Solid Edge part; units mm, degrees
sketch "Sketch1" plane through (0, 0, 0) normal (0, 0, 1) x (1, 0, 0)
  line L0 (-12.6, 6) -> (13.6, 6)
  line L1 (13.6, 6) -> (13.6, 5)
  line L2 (13.6, 5) -> (12.6, 5)
  line L3 (12.6, 5) -> (12.6, -5)
  line L4 (12.6, -5) -> (13.6, -5)
  line L5 (13.6, -5) -> (13.6, -6)
  line L6 (13.6, -6) -> (12.6, -6)
  line L7 (12.6, -6) -> (-12.6, -6)
  line L8 (-12.6, -6) -> (-12.6, 6)
  dimension "D1" = 13.6
  dimension "D2" = 12.6
  dimension "D3" = 12.6
extrude "Protrusion1" add sketch "Sketch1" along normal mid plane 10
sketch "Sketch2" plane through (-12.6, 0, 0) normal (-1, 0, 0) x (0, -1, 0)
  line L0 (-1.118, 1) -> (1.118, 1)
  arc A0 (1.118, 1) -> (-1.118, 1) centre (0, 0) cw
extrude "Extrusionsausprägung_2" add sketch "Sketch2" along normal blind 10
sketch "Sketch3" plane through (0.5, -6, 0) normal (0, -1, 0) x (1, 0, 0)
  line L0 (12.1, 5) -> (12.1, 0.5)
  line L1 (12.1, 0.5) -> (14.7225, 0.5)
  line L2 (14.7225, 0.5) -> (14.7225, -0.5)
  line L3 (14.7225, -0.5) -> (12.1, -0.5)
  line L4 (12.1, -0.5) -> (12.1, -5)
  line L5 (12.1, -5) -> (16.9728, -5)
  line L6 (16.9728, -5) -> (16.9728, 5)
  line L7 (16.9728, 5) -> (12.1, 5)
  dimension "D1" = 14.7225
extrude "Extrusionsausschnitt_1" cut sketch "Sketch3" against normal blind 24
Part model, mm, in its own coordinate system. A direction names the side the tool comes from. Coordinates: 2 decimals unless noted, no trailing zeros. Order: outer loops, then holes, each group sorted by start corner. A loop starts at its lowest first (then second) coordinate and runs counter-clockwise, first axis right, second up. Notation, with made-up numbers: M 62.5,33.5 L 97.5,33.5 A31 ccw 97.5,58.5 Z; hole C 27,37 d11. An arc over 180 degrees is marked long. Use a Markdown table: item, result.
(1) Flat gauge pins, fed straight in: pin 1 (3 mm diameter, centred on y = 0, z = -2, fed in from +X); pin 2 (4 mm diameter, centred on x = -15, z = -1, fed in from +Y); pin 3 (0.7 mm diameter, centred on x = -17, y = 0, fed in from +Z). Where does each tip first touch, or does it go through?
A:
| item | result |
|---|---|
| pin 1 | stops at x = 12.6 |
| pin 2 | stops at y = 1.5 |
| pin 3 | stops at z = 1 |
(2) Cut at A-A on z = 0. Write the cut outline in (x, y).
A:
| item | result |
|---|---|
| outline | M -22.6,-1.5 L -12.6,-1.5 L -12.6,-6 L 13.6,-6 L 13.6,-5 L 12.6,-5 L 12.6,5 L 13.6,5 L 13.6,6 L -12.6,6 L -12.6,1.5 L -22.6,1.5 Z |
(3) Probe L1, parallel to X at y = 1, z = -1; L2, parallel to X at y = -3.25, z = 3.25; L3, parallel to Z at x = -20, y = -0.5. List the from-to ranges inside material, lowest first.
A:
| item | result |
|---|---|
| L1 | x = -22.6 to 12.6 |
| L2 | x = -12.6 to 12.6 |
| L3 | z = -1.41 to 1 |
(4) Cut at B-B on y = 0. Write the cut outline in (x, z).
A:
| item | result |
|---|---|
| outline | M -22.6,-1.5 L -12.6,-1.5 L -12.6,-5 L 12.6,-5 L 12.6,5 L -12.6,5 L -12.6,1 L -22.6,1 Z |
(5) Cut at D-D on z = 1.5. Write the cut outline in (x, y), then the cut area to 3 significant figures.
A:
| item | result |
|---|---|
| outline | M -12.6,-6 L 12.6,-6 L 12.6,6 L -12.6,6 Z |
| area | 302 mm^2 |
(6) Pull direction Y, two halves, no side cores. Call faces 5 (the flat face through (0, 0, 5)), 6 (the flat face through (0, 6, 0)), 7 (the flat face through (13, 5, 0)): released by +Y, released by -Y, zero draft, split by the parting line, or undercut.
A:
| item | result |
|---|---|
| face 5 | zero draft |
| face 6 | released by +Y |
| face 7 | undercut |
(7) Cut at C-C on y = -4.25. Write the cut outline in (x, z), then the cut area to 3 significant figures.
A:
| item | result |
|---|---|
| outline | M -12.6,-5 L 12.6,-5 L 12.6,5 L -12.6,5 Z |
| area | 252 mm^2 |
(8) Tool access for faces 1 (the flat face through (-18, 0, 1)), 2 (the cylindrical face through (-17.5, 0, -1.5)), 3 (the flat face through (13.1, 5.5, -0.5)), 4 (the flat face through (13.1, 5.5, 0.5)): list every direction of +Z, -Z, +X, -X, +Y, -Y with a clear straight run to the whole face (end or side of a thin tool).
A:
| item | result |
|---|---|
| face 1 | +Z, -X, +Y, -Y |
| face 2 | -X |
| face 3 | -Z, +X, +Y, -Y |
| face 4 | +Z, +X, +Y, -Y |
